Geometry: see drawing. Coordinates: mm, zero at the bounding-box minimum. Give positions to 0.01 mm unless a question says otherwise; leave off trailing zeros. Order: outer loops, then holes, each group sorted by start corner. A loop starts at its lowest first (then second) coordinate and runs counter-clockwise, first axis right, second up. Notation, with made-up numbers: (46.25, -25) - (51.25, -25) arc R22 ccw to (51.25, -7) - close; hole circle Ø8 at (28, 61.5). An arc over 180 degrees is marked (long way). One line per question, with ' | ' between items. Start each with the question number.
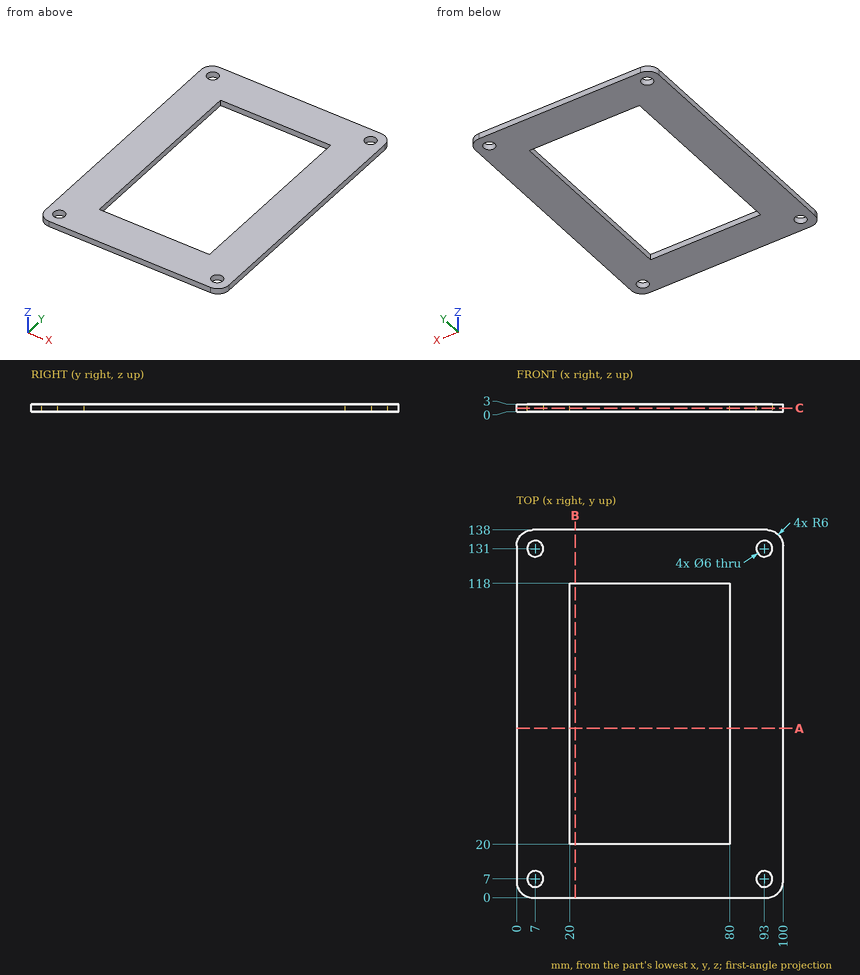
(1) Cut plane C-C, the plane z = 1.45. Return the cut outline in (x, y), plus the area to 3 significant figures.
(2) Cut plane B-B, the plane x = 22. Return the cut outline in (y, z), plus the area to 3 significant figures.
(3) Cut plane A-A, the plane y = 63.5. Return the cut outline in (x, z), plus the area to 3 significant figures.
(4) Material intervals for line 1 along X through (y, z) = (131, 1.65); line 2 along X through (y, z) = (89, 2); line 3 along Y through (x, z) = (26, 0.8), sorted ascending. Write a range as from..to.
Results are:
1) outline: (0, 6) arc R6 ccw to (6, 0) - (94, 0) arc R6 ccw to (100, 6) - (100, 132) arc R6 ccw to (94, 138) - (6, 138) arc R6 ccw to (0, 132) - close; hole circle Ø6 at (7, 7); hole circle Ø6 at (7, 131); hole (20, 20) - (80, 20) - (80, 118) - (20, 118) - close; hole circle Ø6 at (93, 7); hole circle Ø6 at (93, 131) | area: 7,780 mm2
2) outline: (0, 0) - (20, 0) - (20, 3) - (0, 3) - close; (118, 0) - (138, 0) - (138, 3) - (118, 3) - close | area: 120 mm2
3) outline: (0, 0) - (20, 0) - (20, 3) - (0, 3) - close; (80, 0) - (100, 0) - (100, 3) - (80, 3) - close | area: 120 mm2
4) line 1: 0..4, 10..90, 96..100 | line 2: 0..20, 80..100 | line 3: 0..20, 118..138
